For this review, take the finished solid that the model builds, in its own axes (mm). Face numbers are marked on the shaded views. A direction names the side the tool comes from. Coordinates: 2 decimals unless noted, no trailing zeros. Order: outer loops, then holes, each group sorted by start corner. A loop starts at its lowest first (then second) coordinate and runs counter-clockwise, first axis right, second up. Notation, with made-up numbers: (7.25, 63) -> (12.25, 63) arc R11 cw to (12.25, 82) -> close; hole circle Ø3 at (65, -30). An arc over 180 degrees is marked (long way). Write item = value, one per line. Start each with the question number.
1) Consider section C-C on y = 1889.5. Give the boundary of the cut face in (x, z) (3 decimals).
2) Consider section A-A on x = 0. Give the boundary of the cut face in (y, z) (3 decimals).
3) Wall thickness on probe 1 along Y at (x, z) = (-103.5, -1062.5); probe 2 along X at (y, z) = (1724, -1112); probe 3 along Y at (x, z) = (-129, -951): over which ranges is each line inside the solid? List them lowest first. Write a range as [from, to].
4) Consider section D-D on y = 173.5. Give the boundary of the cut face in (x, z) (3 decimals), and give its area (3 significant figures).
5) Machinability: for the marked faces 1, 2, 3, 4 and 5, which of the approach directions +Z, -Z, +X, -X, +Y, -Y give a long, thin tool a straight path to every point of the face, cutting with its end or side? Answer none if there is none.
6) Consider section B-B on z = -1019. Give the boundary of the cut face in (x, y), and give its area (3 significant figures).
7) Insertion check: pin 1 Ø6 at (y, z) = (1670.5, -1003) entering from +X; pin 2 Ø2 at (y, z) = (746, -1002.5) entering from -X; pin 3 Ø6 at (y, z) = (1788, -955) entering from +X. Each pin has a flat end and moves straight along its axis. Give the tip position at first contact, or say it passes through.
8) Draft analysis for pull direction Y (two halves, no side actions). For the marked faces 6, 7 and 8, state which applies: +Y half, -Y half, draft (parallel to the pull), parting line (faces both ways), or undercut.
Autodesk Inventor part; units mm, degrees
ref_plane "Work Plane3" through (121.9127, 0, -1116.765) normal (-1, 0, 0) x (0, 0, 1)
ref_plane "YZ Plane" through (0, 0, 0) normal (1, 0, 0) x (0, 1, 0)
ref_plane "XY Plane" through (0, 0, 0) normal (0, 0, 1) x (1, 0, 0)
sketch "Sketch1" plane through (0, 0, 0) normal (0, 1, 0) x (-1, 0, 0)
  line L0 (117.0873, -996.765) -> (117.0873, -877.765)
  line L1 (-121.9127, -877.765) -> (-121.9127, -996.765)
  line L2 (-121.9127, -1116.765) -> (-1.9127, -1116.765)
  line L3 (-2.9127, -1116.765) -> (117.0873, -1116.765)
  line L4 (117.0873, -996.765) -> (117.0873, -1116.765)
  line L5 (-121.9127, -996.765) -> (-121.9127, -1116.765)
  line L6 (117.0873, -1116.765) -> (-121.9127, -1116.765)
  line L7 (-121.9127, -1116.765) -> (-121.9127, -877.765)
  line L8 (-121.9127, -877.765) -> (117.0873, -877.765)
  line L9 (117.0873, -877.765) -> (117.0873, -1116.765)
  dimension "d0" = 239
ref_plane "Work Plane3" through (121.9127, 0, -1116.765) normal (-1, 0, 0) x (0, 0, 1)
ref_plane "Work Plane2" through (0, 0, 0) normal (0, 1, 0) x (-1, 0, 0)
sketch "Sketch2" plane through (121.9127, 0, -1116.765) normal (-1, 0, 0) x (0, 0, 1)
  line L0 (0, 0) -> (0, 3000)
  line L1 (239, 0) -> (239, 3000)
  line L2 (0, 0) -> (239, 86.9889)
  line L3 (0, 0) -> (254.3385, 0) construction
  line L4 (0, 0) -> (0, 250)
  line L5 (0, 250) -> (239, 250)
  line L6 (239, 250) -> (239, 86.9889)
  point P0 (1116.765, 0)
  dimension "d4" = 3000
  dimension "d5" = 3000
  dimension "d6" = 20
  dimension "d7" = 250
extrude "Extrusion1" add sketch "Sketch2" along normal blind 239
sketch "Sketch3" plane through (121.9127, 250, -877.765) normal (0, 1, 0) x (1, 0, 0)
  circle A0 centre (-121.9127, 119.5) radius 100
  point P0 (-121.9127, -877.765)
  dimension "d10" = 200
extrude "Extrusion2" add sketch "Sketch3" along normal blind 1431
sketch "Sketch4" plane through (0, 1681, -997.265) normal (0, 1, 0) x (1, 0, 0)
  line L0 (-125, -125) -> (125, -125)
  line L1 (125, -125) -> (125, 125)
  line L2 (125, 125) -> (-125, 125)
  line L3 (-125, 125) -> (-125, -125)
  line L4 (-125, -125) -> (125, 125) construction
  line L5 (125, -125) -> (-125, 125) construction
  point P0 (0, -997.265)
  point P1 (0, 0)
  point P2 (0, 0)
  point P3 (0, 0)
  dimension "d13" = 250
  dimension "d14" = 250
extrude "Extrusion3" add sketch "Sketch4" along normal blind 380
sketch "Sketch5" plane through (0, 2061, -997.265) normal (0, 1, 0) x (1, 0, 0)
  line L0 (130, -130) -> (-130, -130)
  line L1 (-130, -130) -> (-130, 130)
  line L2 (-130, 130) -> (130, 130)
  line L3 (130, 130) -> (130, -130)
  line L4 (130, -130) -> (-130, 130) construction
  line L5 (-130, -130) -> (130, 130) construction
  point P0 (0, -997.265)
  point P1 (0, 0)
  point P2 (0, 0)
  dimension "d17" = 260
  dimension "d18" = 260
extrude "Extrusion4" add sketch "Sketch5" along normal blind 20 draft 30
properties part number "side_pillar_01" material "Wood (Maple)"
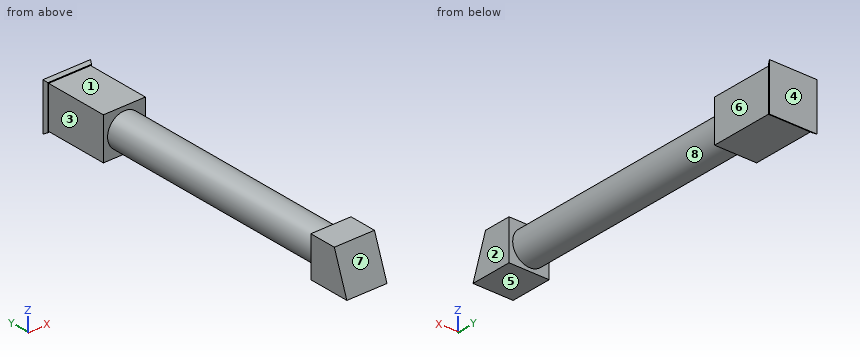
Answer sheet:
q1.outline = (-125, -1122.265) -> (125, -1122.265) -> (125, -872.265) -> (-125, -872.265) -> close
q2.outline = (0, -1116.765) -> (250, -1116.765) -> (250, -1097.265) -> (1681, -1097.265) -> (1681, -1122.265) -> (2061, -1122.265) -> (2061, -1127.265) -> (2081, -1138.812) -> (2081, -855.718) -> (2061, -867.265) -> (2061, -872.265) -> (1681, -872.265) -> (1681, -897.265) -> (250, -897.265) -> (250, -877.765) -> (86.989, -877.765) -> close
q3.probe_1 = [19.75, 250], [1681, 2081]
q3.probe_2 = [-125, 125]
q3.probe_3 = [2061, 2081]
q4.outline = (-117.087, -1116.765) -> (121.913, -1116.765) -> (121.913, -877.765) -> (-117.087, -877.765) -> close
q4.area = 57,100 mm2
q5.face_1 = +Z, +X, -X, -Y
q5.face_2 = +Z, -Z, +X, -Y
q5.face_3 = +Z, -Z, -X, -Y
q5.face_4 = +Z, -Z, +X, -X, +Y
q5.face_5 = -Z, +X, -X, -Y
q6.outline = (-141.55, 2081) -> (-130, 2061) -> (-125, 2061) -> (-125, 1681) -> (-97.61, 1681) -> (-97.61, 250) -> (-117.09, 250) -> (-117.09, 35.58) -> (121.91, 35.58) -> (121.91, 250) -> (97.61, 250) -> (97.61, 1681) -> (125, 1681) -> (125, 2061) -> (130, 2061) -> (141.55, 2081) -> close
q6.area = 431,000 mm2
q7.pin_1 = 99.96
q7.pin_2 = -99.91
q7.pin_3 = 125
q8.face_6 = draft
q8.face_7 = -Y half
q8.face_8 = undercut
